Source: three-view drawing plus pictorial views. Frame: mm from the lowest corner of the part. Give positions to 0.01 mm unless a question says otherwise; leave off trailing zeros. Loops run counter-clockwise (first coordinate to the right, second up) from the corner with the lowest first, then second, coordinate; pieces in that order, holes last. Notation, with made-up numbers: M -13,-33.5 L 0,-33.5 A23 ccw 0,5.5 Z; hole C -32,25 d4. An arc over 180 degrees is marked long. One line per item, written item: value. Start each with the question number.
(1) Pull-direction query (Y, two-part tool) for the marked faces 1, 2 and 3; classes: released by +Y, released by -Y, zero draft, split by the parting line, or undercut.
(2) Pin query (flat end, axial travel): P1, Ø3.5, axis at x = 5.5, y = 6.5, coming from the +Z side. Return the tip coordinate at first contact, or that it passes through.
(3) Section A-A on x = 5. Output: boundary loops of the cut face in (y, z), plus the area to 3 significant figures.
(4) Ray query, line 1 along Y through (x, z) = (5, 23.75); line 2 along Y through (x, z) = (5, 9.75); line 3 along Z through (x, y) = (3.5, 2.75). Return the intervals inside material, ascending. Write a range as from..to.
(5) Section D-D on x = 7.25. Output: boundary loops of the cut face in (y, z).
(6) Section C-C on z = 17.25. Output: boundary loops of the cut face in (x, y).
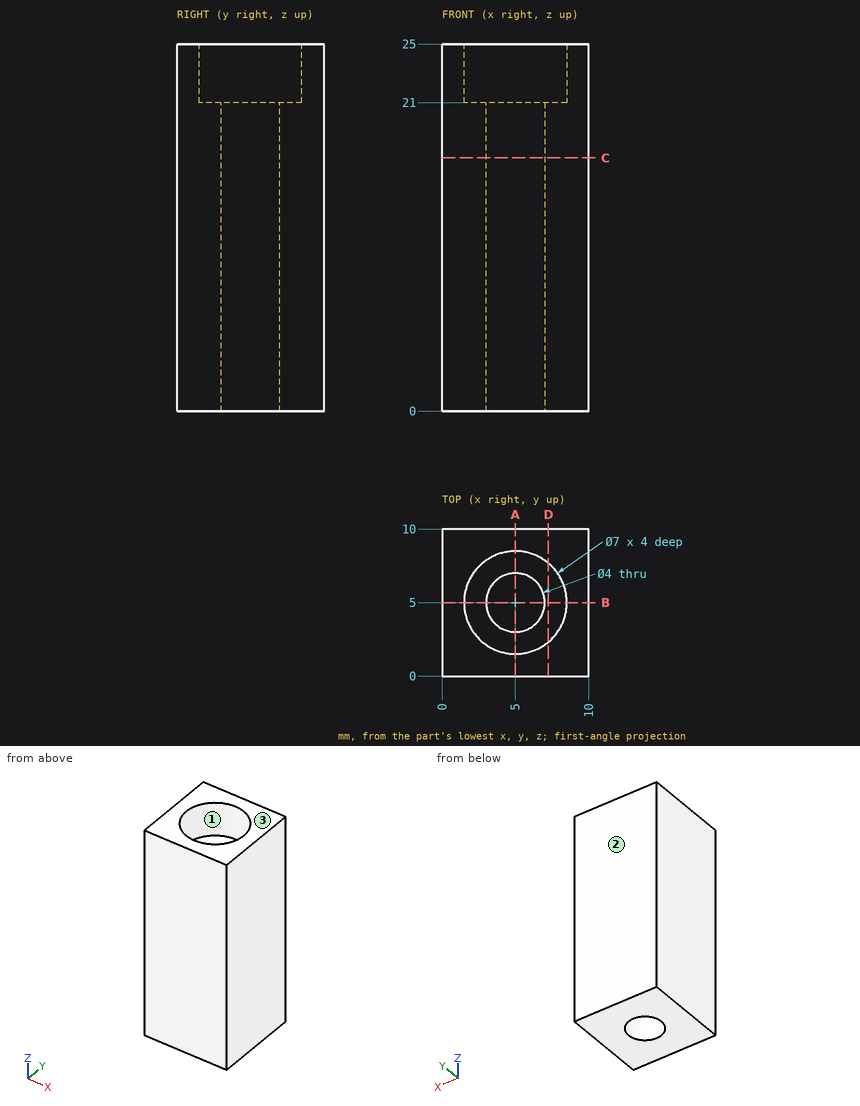
Output values:
1. face 1: undercut
1. face 2: released by +Y
1. face 3: zero draft
2. P1: stops at z = 21
3. outline: M 0,0 L 3,0 L 3,21 L 1.5,21 L 1.5,25 L 0,25 Z; M 7,0 L 10,0 L 10,25 L 8.5,25 L 8.5,21 L 7,21 Z
3. area: 138 mm²
4. line 1: y = 0..1.5, 8.5..10
4. line 2: y = 0..3, 7..10
4. line 3: z = 0..21
5. outline: M 0,0 L 10,0 L 10,25 L 7.68,25 L 7.68,21 L 2.32,21 L 2.32,25 L 0,25 Z
6. outline: M 0,0 L 10,0 L 10,10 L 0,10 Z; hole C 5,5 d4
